Autodesk Inventor part; units mm, degrees
ref_plane "YZ Plane" through (0, 0, 0) normal (1, 0, 0) x (0, 1, 0)
ref_plane "XZ Plane" through (0, 0, 0) normal (0, 1, 0) x (-1, 0, 0)
ref_plane "XY Plane" through (0, 0, 0) normal (0, 0, 1) x (1, 0, 0)
sketch "Sketch1" plane through (0, 0, 0) normal (0, 0, 1) x (1, 0, 0)
  circle A0 centre (0, 0) radius 0.6985
  circle A1 centre (0, 0) radius 1.905
  line L0 (0.6985, 0) -> (7.0485, 0)
  line L1 (7.0485, 0) -> (7.0485, 1.905)
  line L2 (7.0485, 1.905) -> (0.6985, 1.905)
  line L3 (0.6985, 1.905) -> (0.6985, 0)
  point P0 (0.6985, 1.7723)
  point P1 (1.905, 0)
  dimension "d0" = 1.397
  dimension "d1" = 3.81
  dimension "d4" = 6.35
  dimension "d5" = 1.905
extrude "Extrusion1" add sketch "Sketch1" along normal blind 7.62
fillet "Fillet1" radius 3.175 1 edges at (0.6985, 1.7723, 3.81)
fillet "Fillet2" radius 0.5292 1 edges at (1.905, 0, 3.81)
properties part number "innerhinge"
Source: CAD feature listing. Evaluate the final solid. Frame: model axes, mm. A direction names the side the tool comes from. Give positions to 0.01 mm unless a question says otherwise; leave off trailing zeros. Write each loop counter-clockwise with the first axis right and the second up, starting at its lowest first coordinate (ties: lowest second). Pieces come first, ordered by that corner, then holes. Notation, with made-up numbers: (7, 31.5) - (14, 31.5) arc R19 cw to (14, 40.5) - close; hole circle Ø4 at (30.5, 67.25). An arc over 180 degrees is marked (long way). One line per item, written item: value. Start each with the question number.
Q1. First-contact query: pin 1 Ø3.5 at (x, z) = (5, 2.5) entering from -Y. Flat tip, straight axial feed; report the tip coordinate or a pass-through.
Q2. Section query D-D, the plane x = 5.25. Return the cut outline in (y, z) (3 decimals).
Q3. Section query A-A, the plane x = 0. Return the cut outline in (y, z) (1 decimal), then the cut area to 3 significant figures.
Q4. Set-up query: faces 1 (the face through (5, 0, 4)), 2 (the face through (-1.494, -1.182, 3.757)). Return all of +Z, -Z, +X, -X, +Y, -Y with unobstructed straight access to the full face (end or side cutting, diameter ignored); none if empty.
Q5. Material intervals for probe 1 along Y at (x, z) = (0, 3.5) (1 decimal); probe 2 along X at (y, z) = (-0.3, 4.5); probe 3 along Y at (x, z) = (3.5, 0.5) (3 decimals), sorted ascending. Write a range as from..to.
Q6. Section query B-B, the plane y = 0.35. Return the cut outline in (x, z).
Answer:
1. pin 1: stops at y = 0
2. outline: (0, 0) - (1.905, 0) - (1.905, 7.62) - (0, 7.62) - close
3. outline: (-1.9, 0) - (-0.7, 0) - (-0.7, 7.6) - (-1.9, 7.6) - close; (0.7, 0) - (1.9, 0) - (1.9, 7.6) - (0.7, 7.6) - close
3. area: 18.4 mm2
4. face 1: +Z, -Z, +X, -Y
4. face 2: +Z, -Z
5. probe 1: y = -1.9..-0.7, 0.7..1.9
5. probe 2: x = -1.88..-0.63, 0.63..1.9
5. probe 3: y = 0..1.905
6. outline: (-1.87, 0) - (-0.6, 0) - (-0.6, 7.62) - (-1.87, 7.62) - close; (0.6, 0) - (7.05, 0) - (7.05, 7.62) - (0.6, 7.62) - close
